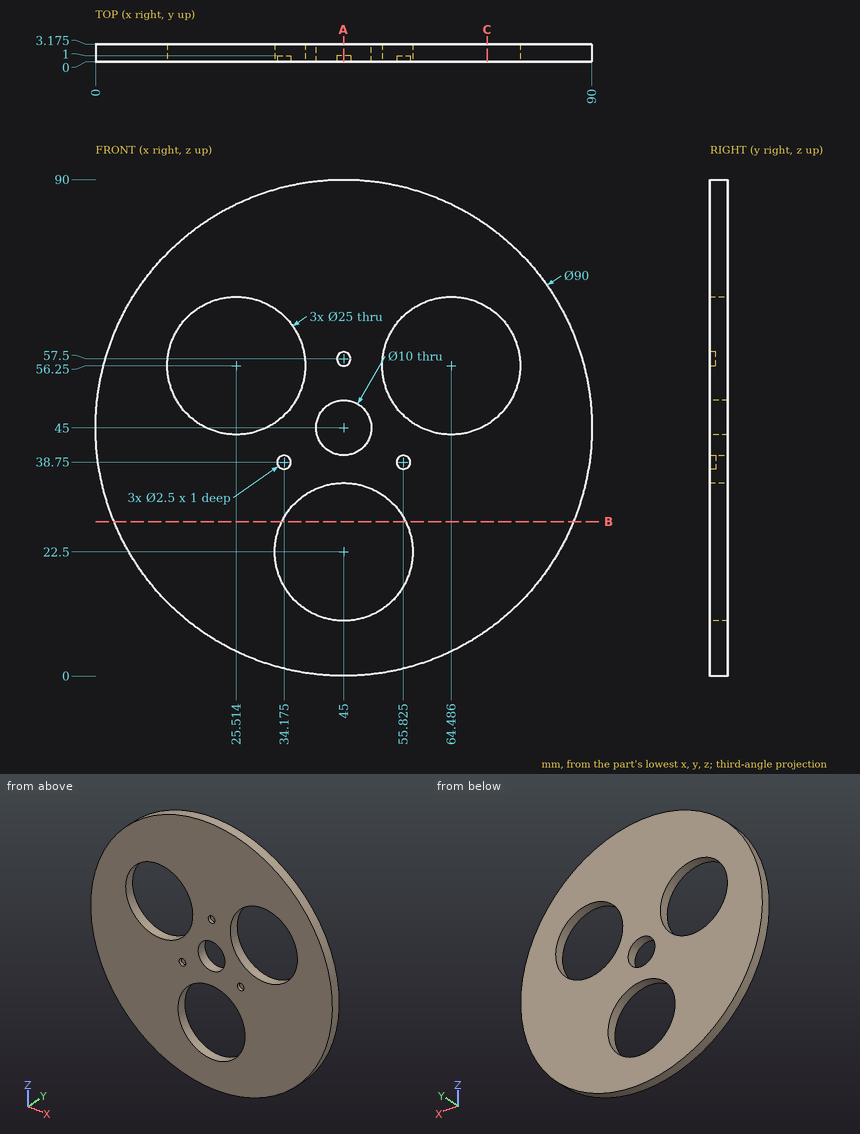
Could you check a few things on this drawing? It's one solid part, dimensions in mm from its lowest x, y, z. Give positions to 0.01 mm unless a question says otherwise; leave off trailing zeros. Write each loop counter-clockwise with the first axis right and the second up, starting at its lowest first coordinate (ties: lowest second). Pieces come first, ordered by that corner, then holes. Notation, with made-up numbers: (84.25, 13.5) -> (102.25, 13.5) arc R7 ccw to (102.25, 18.5) -> close; hole circle Ø2 at (87, 21.5). An arc over 180 degrees is marked (long way). Write item = value, one per line.
(1) Suppose I cut it at B-B on z = 28. Write out the boundary of the cut face in (x, y) (1 decimal), then the cut area to 3 significant figures.
Worked out:
outline = (3.3, 0) -> (33.8, 0) -> (33.8, 3.2) -> (3.3, 3.2) -> close; (56.2, 0) -> (86.7, 0) -> (86.7, 3.2) -> (56.2, 3.2) -> close
area = 193 mm^2
(2) I'm going to push flat-ended pins straight in: P1, Ø1, axis at y = 2.5, z = 24.5, coming from the -X side; P2, Ø1.5, axis at x = 27, y = 2, coming from the +Z side; P3, Ø0.8, axis at x = 34.5, z = 39, coming from the -Y side. Where does each tip first touch, or does it pass through?
Worked out:
P1 = 4.69
P2 = 86.56
P3 = 1
(3) Suppose I cut it at A-A on x = 45. Count the separate pieces of the cut face and the enclosed holes in it, then the cut area to 3 significant figures.
Worked out:
separate_pieces = 3
enclosed_holes = 0
area = 172 mm^2
(4) Suppose I cut it at C-C on x = 71. Write out the boundary of the cut face in (y, z) (1 decimal).
Worked out:
outline = (0, 8.3) -> (3.2, 8.3) -> (3.2, 45.6) -> (0, 45.6) -> close; (0, 66.9) -> (3.2, 66.9) -> (3.2, 81.7) -> (0, 81.7) -> close
(5) I need wall thicknesses on probe 1 along Z at (x, y) = (56, 2.55) (1 decimal); probe 2 along X at (y, z) = (0.5, 52); probe 3 along X at (y, z) = (1.7, 56.25) (1 decimal). Which ranges of each line are inside material? Lowest first, please. Write a range as from..to.
Worked out:
probe_1 = 1.4..16.6, 28.4..47.1, 65.4..88.6
probe_2 = 0.55..13.76, 37.27..52.73, 76.24..89.45
probe_3 = 1.4..13, 38..52, 77..88.6
